Build history of the part. All positions in model axes, mm. Face numbers are marked on the shaded views. A direction names the side the tool comes from. Give positions to 0.01 mm unless a question says otherwise; leave off trailing zeros. Loops run counter-clockwise (first coordinate to the right, second up) from the corner with the lowest first, then second, coordinate; pieces in that order, holes last. Notation, with made-up numbers: (17, 80.5) -> (73, 80.5) arc R21 cw to (73, 110.5) -> close; hole circle Ø1 at (-13, 58.25). An arc over 180 degrees is marked (long way). Answer as a JSON object with one key per item and string values. Group by question number.
Q1. Drop flat-ended pins along their axis: pin 1 (2 mm diameter, centred on x = -9.5, z = -11.5, fed in from -Y); pin 2 (6 mm diameter, centred on y = 11, z = -10, fed in from +X); pin 3 (3 mm diameter, centred on x = 0, y = 15, fed in from +Z); pin 4 (1 mm diameter, centred on y = 9, z = -10, fed in from -X). Give the stop position or say it passes through.
Q2. Band-saw the part on D-D, the plane y = 2. Write the cut outline in (x, z), plus the area to 3 significant figures.
Q3. Wall check: probe 1 along Y at (x, z) = (0, 4.25); probe 2 along X at (y, z) = (13, 4); probe 3 along Y at (x, z) = (0, 3.5). Give the ranges that are in metal, low to high. Write a range as from..to.
Q4. Band-saw the part on A-A, the plane x = 0. Write the cut outline in (y, z), plus the area to 3 significant figures.
Q5. Tool access for the marked faces 1, 2, 3, 4 and 5: list every direction of +Z, -Z, +X, -X, +Y, -Y with a clear straight run to the whole face (end or side of a thin tool).
Q6. Band-saw the part on C-C, the plane z = -8.5. Write the cut outline in (x, y), plus the area to 3 significant figures.
Q7. Band-saw the part on B-B, the plane z = 0.5. Write the cut outline in (x, y).
Q8. Two-plate mould, pull along Y, no slides. Class the marked faces 6, 7, 8 and 9: pulls with the +Y half, pulls with the -Y half, needs draft (parallel to the pull), parting line crosses it, or undercut.
Autodesk Fusion 360 part; units mm, degrees
sketch "Sketch1" plane through (0, 0, 0) normal (1, 0, 0) x (0, 1, 0)
  line L0 (7.7961, -6) -> (22, -6)
  line L1 (8.1, 0) -> (8.1, -8)
  circle A0 centre (0, 0) radius 11.1
  line L2 (0, 11.1) -> (22, 11.1)
  line L3 (22, 11.1) -> (22, -8)
  circle A1 centre (0, 0) radius 8.1
  line L4 (0, 0) -> (-8.1139, 8.1139)
  line L5 (0, 0) -> (-10.06, 4.6911)
  circle A2 centre (0, 0) radius 6.5
  circle A3 centre (0, 0) radius 13.1
  line L6 (-10.06, 4.6911) -> (-10.06, 9.7741)
  line L7 (0, 13.1) -> (22, 13.1)
  line L8 (22, 13.1) -> (22, 11.1)
  line L9 (-9.06, 4.2248) -> (-9.06, 9.7741)
  dimension "d179" = 3
  dimension "d181" = 16.2
  dimension "d182" = 20
  dimension "d6" = 5
  dimension "d33" = 22
extrude "Extrude1" add sketch "Sketch1" along normal mid plane 25 contours L0 L1 A0 A1 L4 | L0 A0 L2 A3 | L0 L2 L3 A3 | A0 A1 L4 L5 L9 | A0 L2 A3 L9 | L2 A3 L7 L8
sketch "Sketch2" plane through (0, 0, -6) normal (0, 0, -1) x (1, 0, 0)
  line L0 (-12.5, -22) -> (12.5, -22)
  line L1 (12.5, -22) -> (12.5, -8.1)
  line L2 (12.5, -8.1) -> (-12.5, -8.1)
  line L3 (-12.5, -8.1) -> (-12.5, -22)
  circle A0 centre (-11.3, 12.8) radius 2.55
  circle A1 centre (-11.3, 12.8) radius 1
  circle A2 centre (4.3, 12.8) radius 2.55
  circle A3 centre (4.3, 12.8) radius 1
  circle A4 centre (0, -13.1) radius 3.2
  circle A5 centre (-7.8, -13.1) radius 2.55
  circle A6 centre (-7.8, -13.1) radius 2.2
  circle A7 centre (7.8, -13.1) radius 2.55
  circle A8 centre (7.8, -13.1) radius 2.2
  dimension "d233" = 2
  dimension "d234" = 2
  dimension "d240" = 15.6
  dimension "d242" = 5.1
  dimension "d243" = 5.1
  dimension "d162" = 6.4
  dimension "d223" = 5.1
  dimension "d224" = 5.1
  dimension "d225" = 4.4
  dimension "d226" = 4.4
  dimension "d227" = 15.6
  dimension "d20" = 7.8
  dimension "d32" = 5
extrude "Extrude2" add sketch "Sketch2" along normal blind 12 contours A5 | A6 | A7 | A8
draft "Draft1" angle 0.5 neutral plane through (0, 11.6452, -6) pull (0, 0, -1) 2 faces at (-5.2532, 13.2271, -14) (10.3468, 13.2271, -14)
sketch "Sketch3" plane through (0, 0, -6) normal (0, 0, -1) x (1, 0, 0)
extrude "Extrude3" cut sketch "Sketch2" against normal blind 20 contours A4
sketch "Sketch4" plane through (0, 0, 13.1) normal (0, 0, 1) x (-1, 0, 0)
  circle A0 centre (0, -13.1) radius 3.2
  line L0 (12.5, 0) -> (-12.5, 0)
  line L1 (-12.5, 0) -> (-12.5, -22)
  line L2 (-12.5, -22) -> (12.5, -22)
  line L3 (12.5, -22) -> (12.5, 0)
  line L4 (3.0022, -18.3) -> (6.0044, -13.1)
  line L5 (6.0044, -13.1) -> (3.0022, -7.9)
  line L6 (3.0022, -7.9) -> (-3.0022, -7.9)
  line L7 (-3.0022, -7.9) -> (-6.0044, -13.1)
  line L8 (-6.0044, -13.1) -> (-3.0022, -18.3)
  line L9 (-3.0022, -18.3) -> (3.0022, -18.3)
  point P0 (0, -13.1)
  dimension "d27" = 5.2
extrude "Extrude4" cut sketch "Sketch4" against normal blind 5 contours L4 L5 L6 L7 L8 L9
chamfer "Chamfer2" distance 2.5 angle 45 7 edges at (-12.5, 22, 3.55) (12.5, 22, 3.55) (0, 22, 13.1) (12.5, 11, 13.1) (12.5, -4.8816, 12.1565) (-12.5, 11, 13.1) (-12.5, -4.8816, 12.1565)
chamfer "Chamfer1" distance 1 angle 45 7 edges at (0, -9.06, 9.4618) (12.5, 13.8, -6) (0, 8.1, -6) (0, 22, -6) (-12.5, 13.8, -6) (11.25, 20.75, -6) (-11.25, 20.75, -6)
chamfer "Chamfer3" distance 0.4 angle 45 6 edges at (4.5033, 15.7, 13.1) (0, 18.3, 13.1) (-4.5033, 15.7, 13.1) (-4.5033, 10.5, 13.1) (0, 7.9, 13.1) (4.5033, 10.5, 13.1)
equation "d20 = d227 / 2"
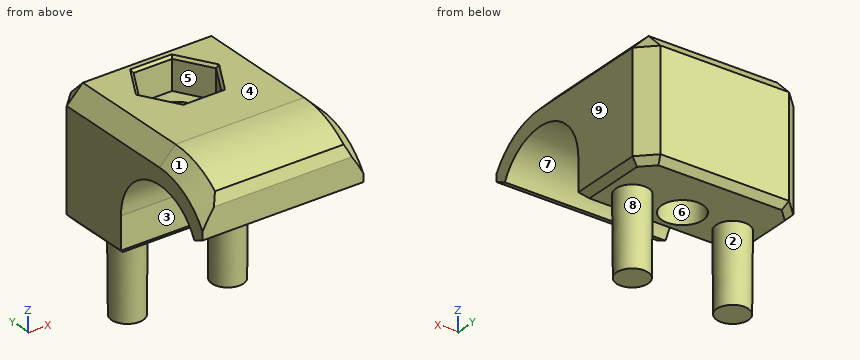
Worked answers:
{
 "1": {"pin 1": "y = 10.7", "pin 2": "x = 10.33", "pin 3": "z = 8.1", "pin 4": "through"},
 "2": {"outline": "(-12.5, 7.85) -> (12.5, 7.85) -> (12.5, 10.6) -> (10, 13.1) -> (-10, 13.1) -> (-12.5, 10.6) -> close", "area": "125 mm2"},
 "3": {"probe 1": "-9.06..-6.9, 6.9..9.9, 16.3..22", "probe 2": "-12.5..-3.2, 3.2..12.5", "probe 3": "-7.51..-7.3, 7.3..9.9, 16.3..22"},
 "4": {"outline": "(-9.06, 4.22) -> (-7.34, 3.42) arc R8.1 cw to (8.1, 0) -> (8.1, -5) -> (9.1, -6) -> (9.9, -6) -> (9.9, 8.1) -> (7.9, 8.1) -> (7.9, 12.7) -> (7.5, 13.1) -> (0, 13.1) arc R13.1 ccw to (-8.31, 10.13) -> (-9.06, 8.46) -> close; (16.3, -6) -> (21, -6) -> (22, -5) -> (22, 10.6) -> (19.5, 13.1) -> (18.7, 13.1) -> (18.3, 12.7) -> (18.3, 8.1) -> (16.3, 8.1) -> close", "area": "225 mm2"},
 "5": {"face 1": "+Z, -X, -Y", "face 2": "-Z", "face 3": "-Z, +X, -X, -Y", "face 4": "+Z, +X, -X, +Y, -Y", "face 5": "+Z"},
 "6": {"outline": "circle Ø5.06 at (-7.8, 13.1); circle Ø5.06 at (7.8, 13.1)", "area": "40.2 mm2"},
 "7": {"outline": "(-12.5, 8.08) -> (12.5, 8.08) -> (12.5, 19.5) -> (10, 22) -> (-10, 22) -> (-12.5, 19.5) -> close; hole circle Ø6.4 at (0, 13.1)"},
 "8": {"face 6": "undercut", "face 7": "undercut", "face 8": "parting line crosses it", "face 9": "needs draft"}
}
